from build123d import *

# Parameters (mm, degrees)
PAD_DEPTH    = 5
SKETCH_R     = 1.75
POCKET_DEPTH = 5


with BuildPart() as part:
    # Sketch001 → Pad (new body)
    with BuildSketch(Plane.YZ):
        with BuildLine():
            Line((39, 9.701271), (39, 40.298729))
            ThreePointArc((39, 40.298729), (38.305966, 42.217718), (36.544988, 43.248811))
            Line((36.544988, 43.248811), (0, 50))
            Line((0, 50), (-36.544988, 43.248811))
            ThreePointArc((-36.544988, 43.248811), (-38.305966, 42.217718), (-39, 40.298729))
            Line((-39, 40.298729), (-39, 9.701271))
            ThreePointArc((-39, 9.701271), (-38.305966, 7.782282), (-36.544988, 6.751189))
            Line((-36.544988, 6.751189), (0, 0))
            Line((0, 0), (36.544988, 6.751189))
            ThreePointArc((36.544988, 6.751189), (38.305966, 7.782282), (39, 9.701271))
        make_face()
    extrude(amount=PAD_DEPTH)

    # Sketch → Pocket (cut)
    with BuildSketch(Plane.YZ):
        with Locations((0, 45)):
            Circle(SKETCH_R)
        with Locations((0, 5)):
            Circle(SKETCH_R)
        with BuildLine():
            Line((-33.75, 10.95), (33.75, 10.95))
            ThreePointArc((33.75, 10.95), (35.517767, 11.682233), (36.25, 13.45))
            Line((36.25, 13.45), (36.25, 36.55))
            ThreePointArc((36.25, 36.55), (35.517767, 38.317767), (33.75, 39.05))
            Line((33.75, 39.05), (-33.75, 39.05))
            ThreePointArc((-33.75, 39.05), (-35.517767, 38.317767), (-36.25, 36.55))
            Line((-36.25, 36.55), (-36.25, 13.45))
            ThreePointArc((-36.25, 13.45), (-35.517767, 11.682233), (-33.75, 10.95))
        make_face()
    extrude(amount=POCKET_DEPTH, mode=Mode.SUBTRACT)


solid = part.part
Check sheet for the modelled part. Datum: model origin and axes. Units: mm. A direction names the side the tool comes from. Round coordinates to 2 decimals unless told otherwise and drop trailing zeros. Order: outer loops, then holes, each group sorted by start corner. A loop starts at its lowest first (then second) coordinate and runs counter-clockwise, first axis right, second up.
Q1. Cross-section at B-B, the plane z = 32.5. Enter the section's corners in (x, y), plus the area to 3 significant figures.
Filled sheet:
outline: (0, -39) - (5, -39) - (5, -36.25) - (0, -36.25) - close; (0, 36.25) - (5, 36.25) - (5, 39) - (0, 39) - close
area: 27.5 mm2
Q2. Depth check by flat-ended pin: P1, Ø2.5, axis at x = 3, y = -3, coming from the -Z side; P2, Ø2, axis at y = 0, z = 45, coming from the -X side. Enter the tip coordinate at first touch or a pass-through.
Filled sheet:
P1: stops at z = 0.32
P2: passes through
Q3. Draft check along Z on faces 1 (the face through (2.465, -38.287, 42.24)), 2 (the face through (2.46, -38.32, 7.8)), 3 (the face through (2.46, -0.38, 43.29)). Enter one of: pulls with the +Z half, pulls with the -Z half, needs draft (parallel to the pull), parting line crosses it, or undercut.
Filled sheet:
face 1: pulls with the +Z half
face 2: pulls with the -Z half
face 3: undercut
Q4. Scan lines: L1, parallel to Z at x = 2.9, y = 0; L2, parallel to Y at x = 4, z = 22; L3, parallel to Z at x = 4.75, y = -1.5. Record each from-to range of solid material in increasing order.
Filled sheet:
L1: z = 0 to 3.25, 6.75 to 10.95, 39.05 to 43.25, 46.75 to 50
L2: y = -39 to -36.25, 36.25 to 39
L3: z = 0.28 to 4.1, 5.9 to 10.95, 39.05 to 44.1, 45.9 to 49.72
Q5. Cross-section at C-C, the plane x = 2.9. Enter the section's corners in (y, z).
Filled sheet:
outline: (-39, 9.7) arc R3 ccw to (-36.54, 6.75) - (0, 0) - (36.54, 6.75) arc R3 ccw to (39, 9.7) - (39, 40.3) arc R3 ccw to (36.54, 43.25) - (0, 50) - (-36.54, 43.25) arc R3 ccw to (-39, 40.3) - close; hole (-36.25, 13.45) arc R2.5 ccw to (-33.75, 10.95) - (33.75, 10.95) arc R2.5 ccw to (36.25, 13.45) - (36.25, 36.55) arc R2.5 ccw to (33.75, 39.05) - (-33.75, 39.05) arc R2.5 ccw to (-36.25, 36.55) - close; hole circle Ø3.5 at (0, 5); hole circle Ø3.5 at (0, 45)
Q6. Set-up check for faces 4 (the face through (2, 0, 10.95)), 5 (the face through (5, 0, 10)): record each of +Z, -Z, +X, -X, +Y, -Y from which the full face is reachable in a straight line by a thin tool's end or side.
Filled sheet:
face 4: +X, -X
face 5: +Z, -Z, +X, +Y, -Y
Q7. Cross-section at A-A, the plane y = 19. Enter the section's corners in (x, z), plus the area to 3 significant figures.
Filled sheet:
outline: (0, 3.51) - (5, 3.51) - (5, 10.95) - (0, 10.95) - close; (0, 39.05) - (5, 39.05) - (5, 46.49) - (0, 46.49) - close
area: 74.4 mm2
